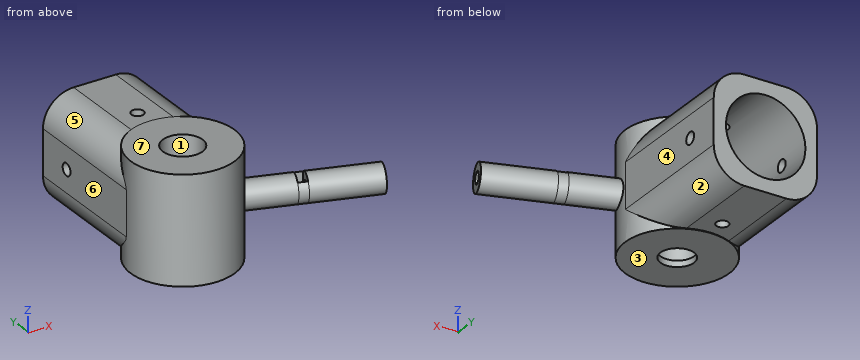
```python
from build123d import *
from build123d.topology import SkipClean

# Parameters (mm, degrees)
SKETCH_1_R                        = 17
SKETCH_1_R_2                      = 6.5
EXTRUDE_2_DEPTH                   = 35
SKETCH_3_W                        = 33.795275063
SKETCH_3_H                        = 34.72803434
SKETCH_3_R                        = 13
EXTRUDE_7_DEPTH                   = 45
SKETCH_4_R                        = 6.5
CUT_EXTRUDE_1_DEPTH               = 60.489495005
SKETCH_12_R                       = 2
CUT_EXTRUDE_11_DEPTH              = 45
SKETCH_15_R                       = 2
CUT_EXTRUDE_12_DEPTH              = 45
FILLET_4_R                        = 10
SKETCH_20_R                       = 13
CUT_EXTRUDE_18_DEPTH              = 31
EXTRUDE_START                     = 1
SKETCH_25_R                       = 13
EXTRUDE_10_DEPTH                  = 1
SKETCH_26_R                       = 6.5
SKETCH_26_R_2                     = 5.5
EXTRUDE_11_DEPTH                  = 2
SKETCH_36_R                       = 4.5
SKETCH_36_R_2                     = 2
EXTRUDE_17_DEPTH                  = 15
EXTRUDE_17_DIRECTION_2_REACH      = 71.637
EXTRUDE_17_DIRECTION_2_END_RADIUS = 17
EXTRUDE_18_DEPTH                  = 3
SKETCH_38_R                       = 4.5
SKETCH_38_R_2                     = 2
EXTRUDE_20_DEPTH                  = 22


with BuildPart() as part:
    # Эскиз1 → Бобышка-Вытянуть2 (new body)
    with BuildSketch(Plane.XY):
        Circle(SKETCH_1_R)
        Circle(SKETCH_1_R_2, mode=Mode.SUBTRACT)
    extrude(amount=EXTRUDE_2_DEPTH)

    # Эскиз3 → Бобышка-Вытянуть7 (add)
    with BuildSketch(Plane(origin=(0, 45, 0), x_dir=(1, 0, 0), z_dir=(0, 1, 0))):
        with Locations((0.102362468, -17.511098906)):
            Rectangle(SKETCH_3_W, SKETCH_3_H)
        with Locations(Location((0, -17.5, 0), (0, 0, 270))):
            Circle(SKETCH_3_R, mode=Mode.SUBTRACT)
    extrude(amount=-EXTRUDE_7_DEPTH)

    # Эскиз4 → Вырез-Вытянуть1 (cut, through all)
    with BuildSketch(Plane(origin=(0, 0, 0), x_dir=(-1, 0, 0), z_dir=(0, 0, -1))):
        with Locations(Location((0, 0, 0), (0, 0, 180))):
            Circle(SKETCH_4_R)
    extrude(amount=-CUT_EXTRUDE_1_DEPTH, mode=Mode.SUBTRACT)

    # Эскиз12 → Вырез-Вытянуть11 (cut)
    with BuildSketch(Plane(origin=(0, 0, 0), x_dir=(-1, 0, 0), z_dir=(0, 0, -1))):
        with Locations((0, 23)):
            Circle(SKETCH_12_R)
    extrude(amount=-CUT_EXTRUDE_11_DEPTH, mode=Mode.SUBTRACT)

    # Эскиз15 → Вырез-Вытянуть12 (cut)
    with BuildSketch(Plane.ZY.offset(16.795275063)):
        with Locations((17.5, 33)):
            Circle(SKETCH_15_R)
    extrude(amount=-CUT_EXTRUDE_12_DEPTH, mode=Mode.SUBTRACT)

    # Скругление4
    # the kernel refuses this fillet: 10 mm, written as the material it takes off along each edge
    with BuildSketch(Plane(origin=(-16.795275063, 70, 34.875116076), x_dir=(1, 0, 0), z_dir=(0, -1, 0))) as fillet_4_piece_1_section:
        with BuildLine():
            CenterArc((FILLET_4_R, -FILLET_4_R), FILLET_4_R, 90, 90)
            Line((0, -FILLET_4_R), (0, 0))
            Line((0, 0), (FILLET_4_R, 0))
        make_face()
    fillet_4_piece_1 = extrude(amount=92.369651061, mode=Mode.PRIVATE)
    fillet_4_piece_1 = fillet_4_piece_1 - Plane(origin=(0, 0, 32.54483178), x_dir=(1, 0, 0), z_dir=(0, 0, -1)) * Cylinder(17, 225, mode=Mode.PRIVATE)
    add(fillet_4_piece_1, mode=Mode.SUBTRACT)
    with BuildSketch(Plane(origin=(17, 70, 0.147081736), x_dir=(0, 0, 1), z_dir=(0, -1, 0))) as fillet_4_piece_2_section:
        with BuildLine():
            CenterArc((FILLET_4_R, FILLET_4_R), FILLET_4_R, 180, 90)
            Line((0, FILLET_4_R), (0, 0))
            Line((0, 0), (FILLET_4_R, 0))
        make_face()
    fillet_4_piece_2 = extrude(amount=95, mode=Mode.PRIVATE)
    fillet_4_piece_2 = fillet_4_piece_2 - Plane(origin=(0, 0, 2.486350956), x_dir=(1, 0, 0), z_dir=(0, 0, -1)) * Cylinder(17, 230, mode=Mode.PRIVATE)
    add(fillet_4_piece_2, mode=Mode.SUBTRACT)
    with BuildSketch(Plane(origin=(17, 70, 34.875116076), x_dir=(0, 0, -1), z_dir=(0, -1, 0))) as fillet_4_piece_3_section:
        with BuildLine():
            CenterArc((FILLET_4_R, -FILLET_4_R), FILLET_4_R, 90, 90)
            Line((0, -FILLET_4_R), (0, 0))
            Line((0, 0), (FILLET_4_R, 0))
        make_face()
    fillet_4_piece_3 = extrude(amount=95, mode=Mode.PRIVATE)
    fillet_4_piece_3 = fillet_4_piece_3 - Plane(origin=(0, 0, 32.535846855), x_dir=(1, 0, 0), z_dir=(0, 0, -1)) * Cylinder(17, 230, mode=Mode.PRIVATE)
    add(fillet_4_piece_3, mode=Mode.SUBTRACT)
    with BuildSketch(Plane(origin=(-16.795275063, 70, 0.147081736), x_dir=(0, 0, 1), z_dir=(0, -1, 0))) as fillet_4_piece_4_section:
        with BuildLine():
            CenterArc((FILLET_4_R, -FILLET_4_R), FILLET_4_R, 90, 90)
            Line((0, -FILLET_4_R), (0, 0))
            Line((0, 0), (FILLET_4_R, 0))
        make_face()
    fillet_4_piece_4 = extrude(amount=92.369651061, mode=Mode.PRIVATE)
    fillet_4_piece_4 = fillet_4_piece_4 - Plane(origin=(0, 0, 2.477367304), x_dir=(1, 0, 0), z_dir=(0, 0, -1)) * Cylinder(17, 225, mode=Mode.PRIVATE)
    add(fillet_4_piece_4, mode=Mode.SUBTRACT)

    # Эскиз20 → Вырез-Вытянуть18 (cut)
    with SkipClean():  # the faces are left unmerged after this step: merging them gives an invalid solid
        with BuildSketch(Plane(origin=(0, 45, 0), x_dir=(1, 0, 0), z_dir=(0, 1, 0))):
            with Locations(Location((0, -17.5, 0), (0, 0, 270))):
                Circle(SKETCH_20_R)
        extrude(amount=-CUT_EXTRUDE_18_DEPTH, mode=Mode.SUBTRACT)

    # Эскиз25 → Бобышка-Вытянуть10 (add)
    with BuildSketch(Plane(origin=(0, 14, 0), x_dir=(1, 0, 0), z_dir=(0, 1, 0)).offset(EXTRUDE_START)):
        with Locations(Location((0, -17.5, 0), (0, 0, 270))):
            Circle(SKETCH_25_R)
    extrude(amount=-EXTRUDE_10_DEPTH)

    # Эскиз26 → Бобышка-Вытянуть11 (add)
    with BuildSketch(Plane(origin=(0, 0, 0), x_dir=(-1, 0, 0), z_dir=(0, 0, -1))):
        Circle(SKETCH_26_R)
        Circle(SKETCH_26_R_2, mode=Mode.SUBTRACT)
    extrude(amount=-EXTRUDE_11_DEPTH)

    # Эскиз36 → Бобышка-Вытянуть17 (add)
    with BuildSketch(Plane(origin=(15.965526333, -5.379751182, 0.007630631), x_dir=(0.001361712962568806, 0.0026227730541390965, -0.9999956333901235), z_dir=(0.9476469847760447, -0.31931956893709296, 0.00045292239977668937))):
        with Locations(Location((-17.511098906, 0, 0), (0, 0, 269.832679764))):
            Circle(SKETCH_36_R)
        with Locations(Location((-17.511098906, 0, 0), (0, 0, 269.832679764))):
            Circle(SKETCH_36_R_2, mode=Mode.SUBTRACT)
    extrude(amount=EXTRUDE_17_DEPTH)

    # Бобышка-Вытянуть17 direction 2: up to this cylinder (the profile starts outside it)
    with SkipClean():  # the faces are left unmerged after this step: merging them gives an invalid solid
        extrude_17_direction_2_end = Plane(origin=(0, 0, 17.518653), z_dir=(0, 0, -1)) * Cylinder(EXTRUDE_17_DIRECTION_2_END_RADIUS, 178.274, mode=Mode.PRIVATE)
        # Эскиз36 → Бобышка-Вытянуть17 direction 2 (add, up to the surface)
        with BuildSketch(Plane(origin=(15.965526333, -5.379751182, 0.007630631), x_dir=(0.001361712962568806, 0.0026227730541390965, -0.9999956333901235), z_dir=(0.9476469847760447, -0.31931956893709296, 0.00045292239977668937)), mode=Mode.PRIVATE) as extrude_17_direction_2_sk1:
            with Locations(Location((-17.511098906, 0, 0), (0, 0, 269.832679764))):
                Circle(SKETCH_36_R)
            with Locations(Location((-17.511098906, 0, 0), (0, 0, 269.832679764))):
                Circle(SKETCH_36_R_2, mode=Mode.SUBTRACT)
        extrude_17_direction_2_tool1 = extrude(extrude_17_direction_2_sk1.sketch, amount=-EXTRUDE_17_DIRECTION_2_REACH, mode=Mode.PRIVATE) - extrude_17_direction_2_end
        add(extrude_17_direction_2_tool1.solids().sort_by_distance((17.337977, -1.281883, 17.518653))[0])
        add(extrude_17_direction_2_tool1.solids().sort_by_distance((17.337977, -1.281883, 17.518653))[1])

    # Эскиз37 → Бобышка-Вытянуть18 (add)
    with SkipClean():  # the faces are left unmerged after this step: merging them gives an invalid solid
        with BuildSketch(Plane(origin=(30.180231104, -10.169544716, 0.014424467), x_dir=(0.00042921059050976356, -0.00014462700029294434, -0.9999998974306447), z_dir=(0.9476469847760448, -0.31931956893709273, 0.0004529223997766894))):
            with BuildLine():
                Line((-19.261024238, 2.979951516), (-20.837057911, 2.979951516))
                ThreePointArc((-20.837057911, 2.979951516), (-13.011024238, -0.051137397), (-20.837057911, -3.08222631))
                Line((-20.837057911, -3.08222631), (-19.261024238, -3.08222631))
                Line((-19.261024238, -3.08222631), (-15.761024238, -3.08222631))
                Line((-15.761024238, -3.08222631), (-14.011024238, -0.051137397))
                Line((-14.011024238, -0.051137397), (-15.761024238, 2.979951516))
                Line((-15.761024238, 2.979951516), (-19.261024238, 2.979951516))
            make_face()
        extrude(amount=EXTRUDE_18_DEPTH)

    # Эскиз38 → Бобышка-Вытянуть20 (add)
    with SkipClean():  # the faces are left unmerged after this step: merging them gives an invalid solid
        with BuildSketch(Plane(origin=(33.023172059, -11.127503423, 0.015783234), x_dir=(0.0004292105905097637, -0.00014462700029294434, -0.9999998974306447), z_dir=(0.9476469847760447, -0.3193195689370928, 0.00045292239977668953))):
            with Locations(Location((-17.511024238, -0.051137397, 0), (0, 0, 270))):
                Circle(SKETCH_38_R)
            with Locations(Location((-17.511024238, -0.051137397, 0), (0, 0, 270))):
                Circle(SKETCH_38_R_2, mode=Mode.SUBTRACT)
        extrude(amount=EXTRUDE_20_DEPTH)


solid = part.part
```
Geometry: final body of the model. Coordinates: model frame, mm. Face numbers are marked on the shaded views. A direction names the side the tool comes from. Coordinates: 2 decimals unless noted, no trailing zeros. Loops run counter-clockwise (first coordinate to the right, second up) from the corner with the lowest first, then second, coordinate; pieces in that order, holes last. Notation, with made-up numbers: (77, 17) -> (115, 17) arc R18 ccw to (115, 34) -> close; hole circle Ø3 at (37, 7). An arc over 180 degrees is marked (long way). Use a Markdown table: item, result. Add a question column.
(1) Access query for the marked faces 4, 5, 6 and 7. Directions: +Z, -Z, +X, -X, +Y, -Y. A direction counts if a zero-diameter tool reaches every point of the face in a straight line with its end or side. Return the directions, or none.
(2) Section query A-A, the plane y = 33. Return loops of the section in (x, z), plus the area to 3 significant figures.
(3) Mould query, pull axis X, two halves, no side actions, for the marked faces 1, 2 and 3. Classes: pulls with the +X half, pulls with the -X half, needs draft (parallel to the pull), parting line crosses it, or undercut.
(4) Line query: line 1 along Y through (x, z) = (0, 12.5); line 2 along Y through (x, z) = (0, 3); line 3 along X through (y, z) = (1, 21). Output: solid intervals per line, ascending.
(5) Section query B-B, the plane x = 0. Return loops of the section in (y, z), plus the area to 3 significant figures.
(6) Section query C-C, the plane y = 18.5. Return loops of the section in (x, z), plus the area to 3 significant figures.
(7) Pin query (flat end, axial travel): pin 1 Ø10.5 at (x, y) = (-0.5, 3) entering from +Z; pin 2 Ø15.5 at (x, z) = (0, 17.5) entering from -Y; pin 3 Ø6.5 at (y, z) = (33, 17.5) entering from -X; pin 4 Ø4 at (y, z) = (-4, 7) entering from -X. Return the tip coordinate at first contact, or that it passes through.
Answer:
| question | item | result |
|---|---|---|
| 1 | face 4 | +Z, -Z, +X, +Y |
| 1 | face 5 | +Z, -X, +Y |
| 1 | face 6 | +Z, -Z, -X, +Y |
| 1 | face 7 | +Z, +X, -X, +Y, -Y |
| 2 | outline | (-16.8, 10.15) arc R10 ccw to (-6.8, 0.15) -> (7, 0.15) arc R10 ccw to (17, 10.15) -> (17, 15.5) -> (12.85, 15.5) arc R13 cw to (-12.85, 15.5) -> (-16.8, 15.5) -> close; (-16.8, 19.5) -> (-12.85, 19.5) arc R13 cw to (12.85, 19.5) -> (17, 19.5) -> (17, 24.88) arc R10 ccw to (7, 34.88) -> (-6.8, 34.88) arc R10 ccw to (-16.8, 24.88) -> close |
| 2 | area | 525 mm^2 |
| 3 | face 1 | undercut |
| 3 | face 2 | pulls with the +X half |
| 3 | face 3 | needs draft |
| 4 | line 1 | y = -17 to -6.5, 6.5 to 15 |
| 4 | line 2 | y = -17 to -6.5, 6.5 to 21, 25 to 45 |
| 4 | line 3 | x = -16.97 to -6.42, 6.42 to 17 |
| 5 | outline | (-17, 0) -> (-5.5, 0) -> (-5.5, 2) -> (-6.5, 2) -> (-6.5, 35) -> (-17, 35) -> close; (5.5, 0) -> (17, 0) -> (17, 0.15) -> (21, 0.15) -> (21, 4.5) -> (15, 4.5) -> (15, 30.5) -> (21, 30.5) -> (21, 34.88) -> (17, 34.88) -> (17, 35) -> (6.5, 35) -> (6.5, 2) -> (5.5, 2) -> close; (25, 0.15) -> (45, 0.15) -> (45, 4.5) -> (25, 4.5) -> close; (25, 30.5) -> (45, 30.5) -> (45, 34.88) -> (25, 34.88) -> close |
| 5 | area | 896 mm^2 |
| 6 | outline | (-16.8, 10.15) arc R10 ccw to (-6.8, 0.15) -> (7, 0.15) arc R10 ccw to (17, 10.15) -> (17, 24.88) arc R10 ccw to (7, 34.88) -> (-6.8, 34.88) arc R10 ccw to (-16.8, 24.88) -> close; hole circle Ø26 at (0, 17.5) |
| 6 | area | 557 mm^2 |
| 7 | pin 1 | stops at z = 35 |
| 7 | pin 2 | stops at y = -17 |
| 7 | pin 3 | stops at x = -16.8 |
| 7 | pin 4 | stops at x = -16.88 |
